from build123d import *

# Parameters (mm, degrees)
F0_W     = 320
F0_H     = 320
F1_DEPTH = 25
F2_ANGLE = 7
F4_DEPTH = 160


with BuildPart() as f1:
    # F0 (on Top) → F1 (new body)
    with BuildSketch(Plane.XY):
        Rectangle(F0_W, F0_H)
    extrude(amount=F1_DEPTH)


with BuildPart() as f1_1:
    # F2: moved
    add(f1.part.rotate(Axis((0, -160, 0), (-1, 0, 0)), F2_ANGLE))

    # F3 (on Right) → F4 (join, symmetric)
    with BuildSketch(Plane.YZ):
        Polygon((157.52013, -39.052658), (-159.990668, 0), (-159.990668, -39.052658), align=None)
    extrude(amount=F4_DEPTH, both=True)


solid = f1_1.part
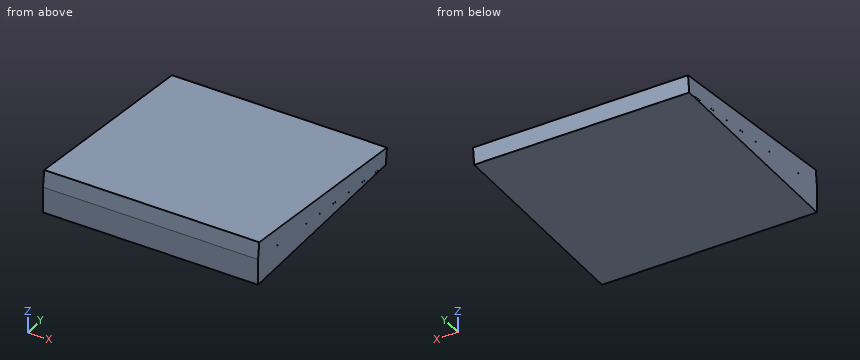
Geometry check sheet. Reference: the model listing, model coordinates, mm. Give positions to 0.01 mm unless a question says otherwise; leave off trailing zeros. Write each loop counter-clockwise with the first axis right and the second up, starting at its lowest first coordinate (ties: lowest second). Pieces come first, ordered by that corner, then holes. Notation, with made-up numbers: M 29,7 L 34,7 A23 ccw 34,35 Z; hole C 17.25,-12 d6. An arc over 180 degrees is marked long. Answer as CSV lines item,"result". Start each with the question number.
Q1. Section check D-D, the plane z = 11.5. Record the cut outline in (x, y), then the cut area to 3 significant figures.
Q2. Section check C-C, the plane z = -7. Record the cut outline in (x, y).
Q3. Go/stop test with flat-tipped pins: pin 1 (1 mm diameter, centred on x = -66, z = -20.5, fed in from -Y); pin 2 (12 mm diameter, centred on x = 66, z = -30.5, fed in from +Y). Record where each tip stops, or that it passes through.
Q4. Section check A-A, the plane y = -1.5. Record the cut outline in (x, z), then the cut area to 3 significant figures.
Geometry says:
1,outline,"M -160,-158.59 L 160,-158.59 L 160,-48.52 L -160,-48.52 Z"
1,area,"35,200 mm^2"
2,outline,"M -160,-159.99 L 160,-159.99 L 160,-103.08 L -160,-103.08 Z; M -160,-102.99 L 160,-102.99 L 160,102.15 L -160,102.15 Z"
3,pin 1,"y = -159.99"
3,pin 2,"y = 159.39"
4,outline,"M -160,-39.05 L 160,-39.05 L 160,-19.49 L -160,-19.49 Z; M -160,-19.46 L 160,-19.46 L 160,5.73 L -160,5.73 Z"
4,area,"14,300 mm^2"
